Check sheet for the drawn part. Datum: minimum x, y, z corner. Units: mm. Coordinates: 2 decimals unless noted, no trailing zeros. Loops run counter-clockwise (first coordinate to the right, second up) from the corner with the lowest first, then second, coordinate; pieces in that order, holes last. Notation, with made-up numbers: M 2,7.25 L 58,7.25 A35 cw 58,42.25 Z; hole C 30,39 d9. An arc over 180 degrees is marked long. Use CSV: the item, a comma, the result in double quotes. Start each with the question number.
(1) Section check B-B on x = 2.5. Record the cut outline in (y, z) (1 decimal).
(2) Section check A-A on z = 9.25. Record the cut outline in (x, y).
(3) Go/stop test with flat-tipped pins: pin 1 Ø5 at (x, z) = (3.5, 5.5) entering from -Y; pin 2 Ø2 at (x, z) = (6.5, 7) entering from -Y; pin 3 Ø2 at (x, y) = (2.5, 3) entering from -Z; pin 4 Ø3 at (y, z) = (6, 7.5) entering from +X. Record where each tip stops, or that it passes through.
(4) Scan lines: line 1 (X direction, y = 1.5, z = 7.5) (1 decimal); line 2 (X direction, y = 3, z = 4.75); line 3 (Y direction, x = 3.5, z = 9) (1 decimal). Record each from-to range of solid material in increasing order.
(5) Section check D-D on z = 2. Record the cut outline in (x, y).
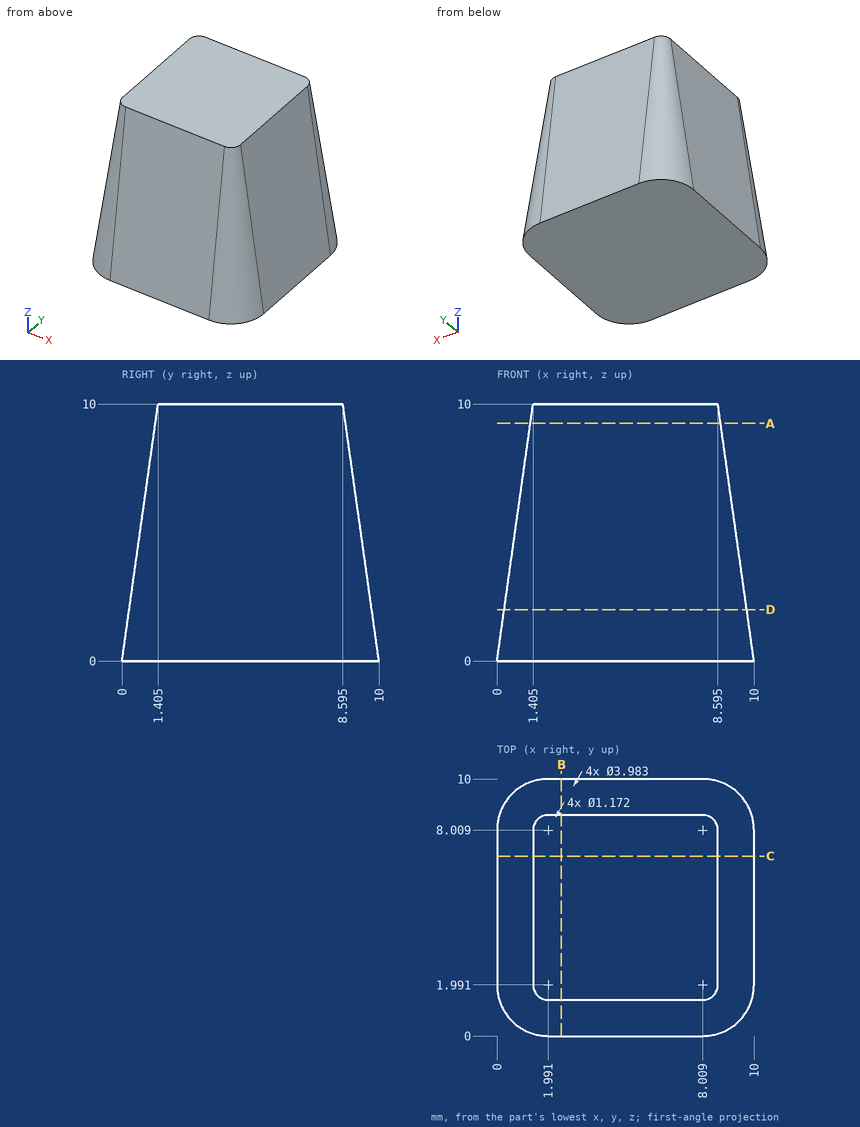
Outcome:
1,outline,"M 0,0 L 10,0 L 8.6,10 L 1.4,10 Z"
2,outline,"M 1.3,1.99 A0.69 ccw 1.99,1.3 L 8.01,1.3 A0.69 ccw 8.7,1.99 L 8.7,8.01 A0.69 ccw 8.01,8.7 L 1.99,8.7 A0.69 ccw 1.3,8.01 Z"
3,pin 1,"stops at y = 0.42"
3,pin 2,"stops at y = 0.84"
3,pin 3,"stops at z = 0"
3,pin 4,"stops at x = 9.16"
4,line 1,"x = 1.2 to 8.8"
4,line 2,"x = 0.67 to 9.33"
4,line 3,"y = 1.3 to 8.7"
5,outline,"M 0.28,1.99 A1.71 ccw 1.99,0.28 L 8.01,0.28 A1.71 ccw 9.72,1.99 L 9.72,8.01 A1.71 ccw 8.01,9.72 L 1.99,9.72 A1.71 ccw 0.28,8.01 Z"
